```python
from build123d import *

# Parameters (mm, degrees)
F1_DEPTH = 63.5
F2_DEPTH = 25.4
F3_DEPTH = 7.9375
F5_R     = 6.35


with BuildPart() as f1:
    # F0 (on Front) → F1 (new body, symmetric)
    with BuildSketch(Plane.XZ):
        Polygon((41.275, -9.525), (41.275, 9.525), (22.225, 9.525), (-41.275, 9.525), (-41.275, -9.525), align=None)
    extrude(amount=F1_DEPTH, both=True)

    # F0 (on Front) → F2 (join, symmetric)
    with BuildSketch(Plane.XZ):
        with BuildLine():
            Line((22.225, 9.525), (41.275, 9.525))
            Line((41.275, 9.525), (41.275, 27.0002))
            ThreePointArc((41.275, 27.0002), (45.9246798487, 38.2255201513), (57.15, 42.8752))
            Line((57.15, 42.8752), (60.325, 42.8752))
            Line((60.325, 42.8752), (60.325, 61.9252))
            Line((60.325, 61.9252), (57.15, 61.9252))
            ThreePointArc((57.15, 61.9252), (32.4542956671, 51.6959043329), (22.225, 27.0002))
            Line((22.225, 27.0002), (22.225, 9.525))
        make_face()
    extrude(amount=F2_DEPTH, both=True)

    # F0 (on Front) → F3 (join, symmetric)
    with BuildSketch(Plane.XZ):
        with BuildLine():
            Line((-41.275, 9.525), (22.225, 9.525))
            Line((22.225, 9.525), (22.225, 27.0002))
            ThreePointArc((22.225, 27.0002), (32.4542956671, 51.6959043329), (57.15, 61.9252))
            add(Edge.make_bspline(
                [(57.15, 61.9252), (4.0777479298, 61.9457326829), (-22.87033014, 33.9522510767), (-41.275, 9.525)],
                knots=[0, 0, 0, 0, 111.5045361635, 111.5045361635, 111.5045361635, 111.5045361635], degree=3))
        make_face()
    extrude(amount=F3_DEPTH, both=True)

    # F0 (on Front) → F4 (revolve)
    with BuildSketch(Plane.XZ):
        Polygon((60.325, 61.9252), (60.325, 42.8752), (85.7335714616, 42.8752), (85.7267106332, 61.9252), align=None)
    revolve(axis=Axis((60.325, 0, 52.3875), (0, 0, 1)))

    # F5
    f5_edges = [f1.edges().sort_by_distance(p)[0] for p in [
        (41.275, -63.5, 0),
        (-41.275, -63.5, 0),
        (-41.275, 63.5, 0),
        (41.275, 63.5, 0),
    ]]
    fillet(f5_edges, radius=F5_R)


solid = f1.part
```
Build history of the part. All positions in model axes, mm. A direction names the side the tool comes from. Give positions to 0.01 mm unless a question says otherwise; leave off trailing zeros. Loops run counter-clockwise (first coordinate to the right, second up) from the corner with the lowest first, then second, coordinate; pieces in that order, holes last.
1) Band-saw the part on A-A on z = -3. List the corners of the cut face in (x, y) (3 decimals).
Values follow:
outline: (-41.275, -57.15) arc R6.35 ccw to (-34.925, -63.5) - (34.925, -63.5) arc R6.35 ccw to (41.275, -57.15) - (41.275, 57.15) arc R6.35 ccw to (34.925, 63.5) - (-34.925, 63.5) arc R6.35 ccw to (-41.275, 57.15) - close
2) Drop flat-ended pins along their axis: P1, Ø5, axis at y = -17, z = 15, coming from the -X side (3 decimals); P2, Ø2, axis at y = -22.5, z = 17.5, coming from the +X side (3 decimals); P3, Ø15, axis at x = 8.5, z = 41.5, coming from the -Y side. Give the stop position or say it passes through.
Values follow:
P1: stops at x = 22.225
P2: stops at x = 41.275
P3: stops at y = -7.94
3) Band-saw the part on B-B on y = -34. List the corners of the cut face in (x, z) (3 decimals), then the cut area to 3 significant figures.
Values follow:
outline: (-41.275, -9.525) - (41.275, -9.525) - (41.275, 9.525) - (-41.275, 9.525) - close
area: 1,570 mm2
4) 3-axis set-ups, long thin cutter, end or side, ignore diameter. For faces 1 (the face through (28.763, -16.791, 47.346)), 2 (the face through (28.763, 16.547, 47.346)), 3 (the face through (37, -25.4, 36)): which of +Z, -Z, +X, -X, +Y, -Y reach the whole face in a straight line?
Values follow:
face 1: +Z, -X, -Y
face 2: +Z, -X, +Y
face 3: +Z, +X, -X, -Y
5) Probe line 1 along Y through (x, z) = (13, 42); line 2 along Z through (x, y) = (24.5, 44.5) (3 decimals); line 3 along Z through (x, y) = (65.5, 1). List the from-to ranges inside material, lowest first.
Values follow:
line 1: y = -7.94 to 7.94
line 2: z = -9.525 to 9.525
line 3: z = 42.88 to 61.93
